Here's the drawing with two shaded views (mm, measured from the low corner). I have some questions. A direction names the side the tool comes from. Coordinates: 2 decimals unless noted, no trailing zeros. Loops run counter-clockwise (first coordinate to the right, second up) from the corner with the lowest first, then second, coordinate; pieces in that order, holes last. Notation, with made-up numbers: (79.25, 47) -> (99.25, 47) arc R11 cw to (99.25, 67) -> close; hole circle Ø7 at (56, 77.5). An arc over 180 degrees is marked (long way). Answer as a JSON object with one key per item and string values. Group by question number.
1) Which directions (+Z, -Z, +X, -X, +Y, -Y) give clear straight access to the entire face, cutting with the end or side of a thin tool? Please do the marked faces 1 and 2.
2) I need wall thicknesses on probe 1 along Y at (x, z) = (79.25, 6.35); probe 2 along Z at (x, y) = (12.7, 4.75); probe 3 along X at (y, z) = (84.5, 1.75). Which ranges of each line are inside material? Lowest first, please. Write a range as [from, to].
3) I want a section at A-A (y = 106). Write out the boundary of the cut face in (x, z), then the cut area to 3 significant figures.
4) I'm going to push flat-ended pins straight in: pin 1 (3 mm diameter, centred on y = 172.72, z = 6.35, fed in from +X); pin 2 (4 mm diameter, centred on x = 23.5, z = 10, fed in from +Y); pin 3 (6 mm diameter, centred on x = 12.7, z = 6.35, fed in from +Y). Where does each tip first touch, or does it pass through?
5) I want a section at B-B (y = 140). Write out the boundary of the cut face in (x, z), then the cut area to 3 significant figures.
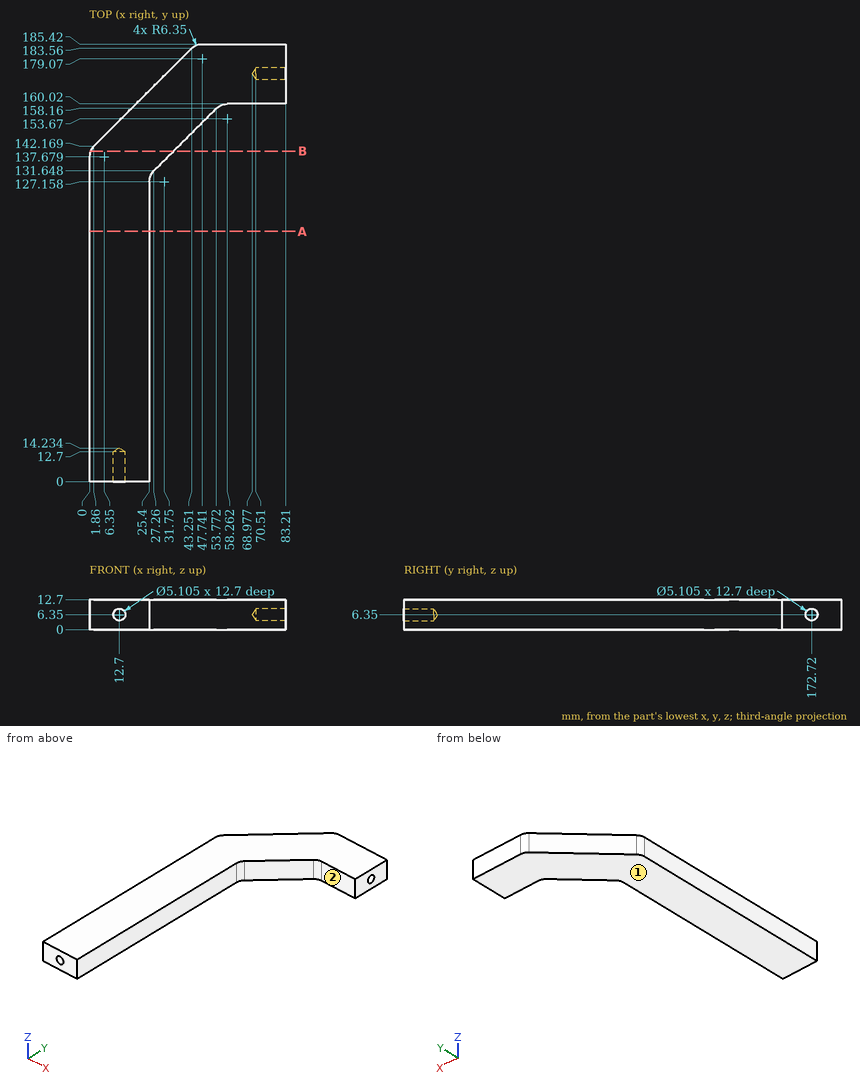
Determined:
{
 "1": {"face 1": "-Z, +X, -X, +Y, -Y", "face 2": "+Z, -Z, +X, -Y"},
 "2": {"probe 1": "[160.02, 170.17], [175.27, 185.42]", "probe 2": "[0, 3.8], [8.9, 12.7]", "probe 3": "[0, 25.4]"},
 "3": {"outline": "(0, 0) -> (25.4, 0) -> (25.4, 12.7) -> (0, 12.7) -> close", "area": "323 mm^2"},
 "4": {"pin 1": "x = 69.88", "pin 2": "y = 165.81", "pin 3": "y = 156.01"},
 "5": {"outline": "(0.44, 0) -> (35.61, 0) -> (35.61, 12.7) -> (0.44, 12.7) -> close", "area": "447 mm^2"}
}
